Work out the finished part from the listing and answer in its coordinate system (mm). Face numbers are marked on the shaded views. Round coordinates to 2 decimals unless told otherwise and drop trailing zeros. Loops run counter-clockwise (first coordinate to the right, second up) from the corner with the lowest first, then second, coordinate; pieces in that order, holes last. Notation, with made-up numbers: M -35,-23 L 13,-23 A15 ccw 13,-19 Z; hole C 44.5,56.25 d8. An arc over 180 degrees is marked long. One line per item, written item: value.
```python
from build123d import *

# Parameters (mm, degrees)
F0_R     = 17.5
F0_R_2   = 7.25
F1_DEPTH = 2
F2_R     = 8.75
F2_R_2   = 7.25
F3_DEPTH = 5
F2_R_3   = 17.5
F2_R_4   = 16
F4_DEPTH = 25
F5_W     = 8.5
F5_H     = 17.5
F6_DEPTH = 27.001


with BuildPart() as f1:
    # F0 (on Top) → F1 (new body)
    with BuildSketch(Plane.XY):
        Circle(F0_R)
        Circle(F0_R_2, mode=Mode.SUBTRACT)
    extrude(amount=F1_DEPTH)

    # F2 (on face) → F3 (join)
    with BuildSketch(Plane.XY.offset(2)):
        Circle(F2_R)
        Circle(F2_R_2, mode=Mode.SUBTRACT)
    extrude(amount=F3_DEPTH)

    # F2 (on face) → F4 (join)
    with BuildSketch(Plane.XY.offset(2)):
        Circle(F2_R_3)
        Circle(F2_R_4, mode=Mode.SUBTRACT)
    extrude(amount=F4_DEPTH)

    # F5 (on Top) → F6 (cut, through all)
    with BuildSketch(Plane.XY):
        with Locations((0, 8.75)):
            Rectangle(F5_W, F5_H)
    extrude(amount=F6_DEPTH, mode=Mode.SUBTRACT)


solid = f1.part
```
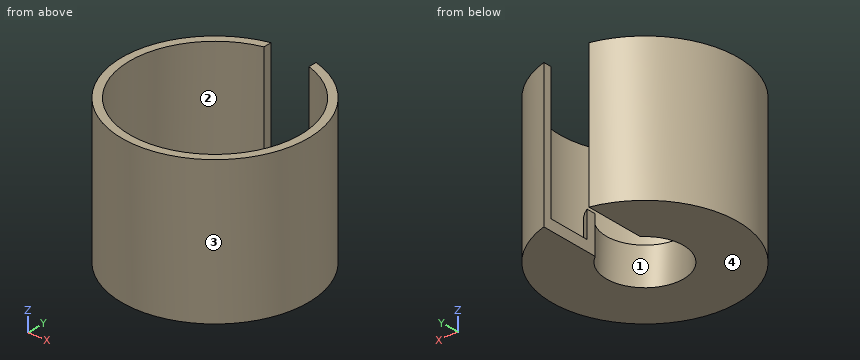
1) Find section C-C (x = -5). Give the vertices of the cut face in (y, z).
Check values:
outline: M -16.77,0 L -5.25,0 L -5.25,7 L -7.18,7 L -7.18,2 L -15.2,2 L -15.2,27 L -16.77,27 Z; M 5.25,0 L 16.77,0 L 16.77,27 L 15.2,27 L 15.2,2 L 7.18,2 L 7.18,7 L 5.25,7 Z
2) Find section A-A (y = 0). Give the vertices of the cut face in (x, z), then the cut area to 3 significant figures.
Check values:
outline: M -17.5,0 L -7.25,0 L -7.25,7 L -8.75,7 L -8.75,2 L -16,2 L -16,27 L -17.5,27 Z; M 7.25,0 L 17.5,0 L 17.5,27 L 16,27 L 16,2 L 8.75,2 L 8.75,7 L 7.25,7 Z
area: 131 mm2
3) Each of these flat-tipped pins is pushed along its axis until it touches: pin 1 (4 mm diameter, centred on x = 0, z = 21, fed in from +Y); pin 2 (1 mm diameter, centred on x = -10.5, z = 13, fed in from +Y); pin 3 (4 mm diameter, centred on y = -6.5, z = 14, fed in from -X). Where does it stop, or does it pass through?
Check values:
pin 1: y = -15.87
pin 2: y = 14.36
pin 3: x = -16.91
4) The mould has two halves that part along Y. Classify the marked faces 1, 2, 3 and 4: +Y half, -Y half, draft (parallel to the pull), parting line (faces both ways), or undercut.
Check values:
face 1: undercut
face 2: undercut
face 3: parting line
face 4: draft
5) Find section D-D (x = 0). Give the vertices of the cut face in (y, z), then the cut area to 3 significant figures.
Check values:
outline: M -17.5,0 L -7.25,0 L -7.25,7 L -8.75,7 L -8.75,2 L -16,2 L -16,27 L -17.5,27 Z
area: 65.5 mm2
6) Find the intervals of material crossed by probe 1 along X at (y, z) = (0, 14.25); probe 2 along Z at (x, y) = (10, 11.5); probe 3 along X at (y, z) = (-11, 9.25), in increasing order. Write a range as from..to.
Check values:
probe 1: -17.5..-16, 16..17.5
probe 2: 0..2
probe 3: -13.61..-11.62, 11.62..13.61
7) Find section B-B (z = 6.5). Give the vertices of the cut face in (x, y).
Check values:
outline: M -4.25,5.87 L -4.25,7.65 A8.75 ccw long 4.25,7.65 L 4.25,5.87 A7.25 cw long Z; M -4.25,15.43 L -4.25,16.98 A17.5 ccw long 4.25,16.98 L 4.25,15.43 A16 cw long Z
